The model under review builds one solid part; all positions refer to its coordinate system, in mm. Face numbers are marked on the shaded views. A direction names the side the tool comes from. Coordinates: 2 decimals unless noted, no trailing zeros. Order: outer loops, then holes, each group sorted by start corner. A loop starts at its lowest first (then second) coordinate and runs counter-clockwise, first axis right, second up. Notation, with made-up numbers: (-18, 27.5) -> (-10, 27.5) arc R12 cw to (-10, 38.5) -> close; hole circle Ø10 at (74, -10.5). An arc over 180 degrees is marked (long way). Use one line per item in the form item = value. Start each with the question number.
(1) Mouldability with a two-part tool opening along Y and no side actions: class the marked faces 3, 4 and 5 as +Y half, -Y half, draft (parallel to the pull), parting line (faces both ways), or undercut.
(2) Take a section at C-C (x = -4.25). State the section outline as (y, z) points, then the cut area to 3 significant figures.
(3) Take a section at D-D (z = 5.75). State the section outline as (x, y) points.
(4) For the marked faces 1 and 2, list the 3-axis set-ups (+Z, -Z, +X, -X, +Y, -Y) from which the entire face can be reached by the end or side of a thin tool; tool diameter is ignored.
(5) Take a section at B-B (z = 2). State the section outline as (x, y) points.
(6) Insertion check: pin 1 Ø1 at (y, z) = (5.5, 2.5) entering from +X; pin 2 Ø10 at (x, y) = (-20, -2.5) entering from +Z; pin 3 Ø0.9 at (x, y) = (-15, -2.5) entering from -Z. Each pin has a flat end and moves straight along its axis. Give the tip position at first contact, or say it passes through.
(7) Take a section at A-A (y = 9.5). State the section outline as (x, z) points.
(8) Wall thickness on line 1 along Y through (x, z) = (-9.75, 0.75); line 2 along Z through (x, y) = (-16.75, -6); line 3 along Z through (x, y) = (-16.25, 4.25): over which ranges is each line inside the solid? List them lowest first.
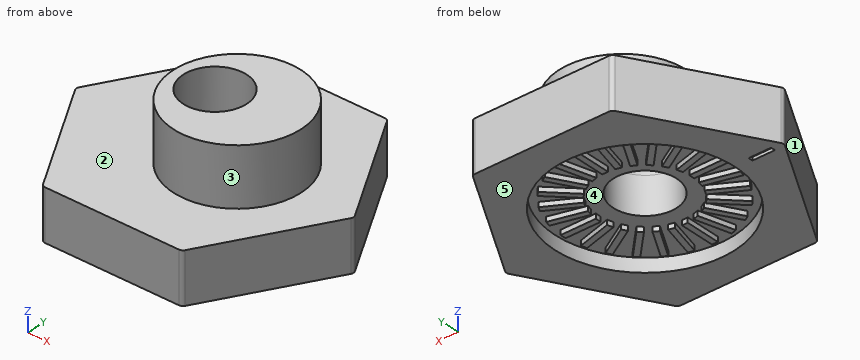
```python
from build123d import *

# Parameters (mm, degrees)
F1_DEPTH  = 4.0132
F2_R      = 2.5146
F3_DEPTH  = 25.4
F4_R      = 5.0673
F4_R_2    = 2.5146
F5_DEPTH  = 4.572
F6_R      = 7.1374
F7_DEPTH  = 1.0922
F8_W      = 2.794
F8_H      = 0.4572
F8_W_2    = 0.4572
F8_H_2    = 2.794
F9_DEPTH  = 0.381
F10_R     = 0.381
F11_W     = 1.778
F11_H     = 0.3556
F12_DEPTH = 0.254


with BuildPart() as f1:
    # F0 (on Top) → F1 (new body)
    with BuildSketch(Plane.XY):
        Polygon((-7.126325, 12.257675), (-18.183506, 12.257675), (-23.712097, 2.681875), (-18.183506, -6.893925), (-7.126325, -6.893925), (-1.597734, 2.681875), align=None)
    extrude(amount=F1_DEPTH)

    # F2 (on face) → F3 (cut)
    with BuildSketch(Plane.XY.offset(4.0132)):
        with Locations((-12.654915, 2.681875)):
            Circle(F2_R)
    extrude(amount=-F3_DEPTH, mode=Mode.SUBTRACT)

    # F4 (on face) → F5 (join)
    with BuildSketch(Plane.XY.offset(4.0132)):
        with Locations((-10.889615, 2.681875)):
            Circle(F4_R)
        with Locations((-12.654915, 2.681875)):
            Circle(F4_R_2, mode=Mode.SUBTRACT)
    extrude(amount=F5_DEPTH)

    # F6 (on face) → F7 (cut)
    with BuildSketch(Plane(origin=(0, 0, 0), x_dir=(1, 0, 0), z_dir=(0, 0, -1))):
        with Locations((-12.654915, -2.681875)):
            Circle(F6_R)
    extrude(amount=-F7_DEPTH, mode=Mode.SUBTRACT)

    # F8 (on face) → F9 (join)
    with BuildSketch(Plane(origin=(0, 0, 1.0922), x_dir=(1, 0, 0), z_dir=(0, 0, -1))):
        with Locations((-7.549515, -2.681875)):
            Rectangle(F8_W, F8_H)
        Polygon((-9.132042, -1.50126), (-9.01371, -1.942881), (-6.314913, -1.21974), (-6.433245, -0.778119), align=None)
        Polygon((-9.557647, -0.629701), (-9.329047, -1.025648), (-6.909372, 0.371352), (-7.137972, 0.767299), align=None)
        Polygon((-10.194325, 0.102005), (-9.871036, -0.221285), (-7.89538, 1.754372), (-8.218669, 2.077661), align=None)
        Polygon((-10.998689, 0.643994), (-10.602742, 0.415394), (-9.205742, 2.835069), (-9.601689, 3.063669), align=None)
        Polygon((-11.915922, 0.959331), (-11.4743, 0.840999), (-10.75116, 3.539795), (-11.192781, 3.658127), align=None)
        with Locations((-12.654915, 2.423525)):
            Rectangle(F8_W_2, F8_H_2)
        Polygon((-13.835531, 0.840999), (-13.393909, 0.959331), (-14.11705, 3.658127), (-14.558671, 3.539795), align=None)
        Polygon((-14.707089, 0.415394), (-14.311142, 0.643994), (-15.708142, 3.063669), (-16.104089, 2.835069), align=None)
        Polygon((-15.438795, -0.221285), (-15.115506, 0.102005), (-17.091162, 2.077661), (-17.414451, 1.754372), align=None)
        Polygon((-15.980784, -1.025648), (-15.752184, -0.629701), (-18.171859, 0.767299), (-18.400459, 0.371352), align=None)
        Polygon((-16.296121, -1.942881), (-16.177789, -1.50126), (-18.876586, -0.778119), (-18.994918, -1.21974), align=None)
        with Locations((-17.760315, -2.681875)):
            Rectangle(F8_W, F8_H)
        Polygon((-16.177789, -3.86249), (-16.296121, -3.420869), (-18.994918, -4.144009), (-18.876586, -4.58563), align=None)
        Polygon((-15.752184, -4.734048), (-15.980784, -4.338101), (-18.400459, -5.735101), (-18.171859, -6.131048), align=None)
        Polygon((-15.115506, -5.465754), (-15.438795, -5.142465), (-17.414451, -7.118121), (-17.091162, -7.44141), align=None)
        Polygon((-14.311142, -6.007743), (-14.707089, -5.779143), (-16.104089, -8.198818), (-15.708142, -8.427418), align=None)
        Polygon((-13.393909, -6.32308), (-13.835531, -6.204748), (-14.558671, -8.903545), (-14.11705, -9.021877), align=None)
        with Locations((-12.654915, -7.787275)):
            Rectangle(F8_W_2, F8_H_2)
        Polygon((-11.4743, -6.204748), (-11.915922, -6.32308), (-11.192781, -9.021877), (-10.75116, -8.903545), align=None)
        Polygon((-10.602742, -5.779143), (-10.998689, -6.007743), (-9.601689, -8.427418), (-9.205742, -8.198818), align=None)
        Polygon((-9.871036, -5.142465), (-10.194325, -5.465754), (-8.218669, -7.44141), (-7.89538, -7.118121), align=None)
        Polygon((-9.329047, -4.338101), (-9.557647, -4.734048), (-7.137972, -6.131048), (-6.909372, -5.735101), align=None)
        Polygon((-9.01371, -3.420869), (-9.132042, -3.86249), (-6.433245, -4.58563), (-6.314913, -4.144009), align=None)
    extrude(amount=F9_DEPTH)

    # F10
    f10_edges = [f1.edges().sort_by_distance(p)[0] for p in [
        (-7.126325, 12.257675, 2.0066),
        (-18.183506, 12.257675, 2.0066),
        (-23.712097, 2.681875, 2.0066),
        (-18.183506, -6.893925, 2.0066),
        (-7.126325, -6.893925, 2.0066),
        (-1.597734, 2.681875, 2.0066),
    ]]
    fillet(f10_edges, radius=F10_R)

    # F11 (on face) → F12 (cut)
    with BuildSketch(Plane(origin=(0, 0, 0), x_dir=(1, 0, 0), z_dir=(0, 0, -1))):
        with Locations((-21.925915, -2.681875)):
            Rectangle(F11_W, F11_H)
    extrude(amount=-F12_DEPTH, mode=Mode.SUBTRACT)


solid = f1.part
```
Findings:
q1.face_3 = parting line
q1.face_4 = undercut
q1.face_5 = draft
q2.outline = (-1.91, 0) -> (7.28, 0) -> (7.28, 4.01) -> (-1.91, 4.01) -> close
q2.area = 36.9 mm²
q3.outline = circle Ø10.13 at (-10.89, 2.68); hole circle Ø5.03 at (-12.65, 2.68)
q4.face_1 = +Z, -Z, -X, -Y
q4.face_2 = +Z
q5.outline = (-23.6, 2.49) -> (-18.29, -6.7) arc R0.38 ccw to (-17.96, -6.89) -> (-7.35, -6.89) arc R0.38 ccw to (-7.02, -6.7) -> (-1.71, 2.49) arc R0.38 ccw to (-1.71, 2.87) -> (-7.02, 12.07) arc R0.38 ccw to (-7.35, 12.26) -> (-17.96, 12.26) arc R0.38 ccw to (-18.29, 12.07) -> (-23.6, 2.87) arc R0.38 ccw to start; hole circle Ø5.03 at (-12.65, 2.68)
q6.pin_1 = -2.94
q6.pin_2 = 4.01
q6.pin_3 = 0.71
q7.outline = (-19.78, 0) -> (-14.77, 0) -> (-14.77, 1.09) -> (-10.54, 1.09) -> (-10.54, 0) -> (-5.53, 0) -> (-5.53, 4.01) -> (-19.78, 4.01) -> close
q8.line_1 = -6.89 to -3.84, -2.81 to -1.89, -0.55 to 0.1, 5.26 to 5.91, 7.26 to 8.17, 9.2 to 12.26
q8.line_2 = 0 to 4.01
q8.line_3 = 1.09 to 4.01
